Source: CAD feature listing. Evaluate the final solid. Frame: model axes, mm. Face numbers are marked on the shaded views. A direction names the side the tool comes from. Round coordinates to 2 decimals unless told otherwise and drop trailing zeros. Order: outer loops, then holes, each group sorted by start corner. A loop starts at its lowest first (then second) coordinate and runs counter-clockwise, first axis right, second up. Notation, with made-up numbers: (29, -19.75) -> (78, -19.75) arc R11 cw to (78, -4.75) -> close; hole circle Ø7 at (-5.5, -16). An arc over 180 degrees is marked (long way). Answer as CSV lines item,"result".
from build123d import *

# Parameters (mm, degrees)
F1_DEPTH = 1.5
F3_DEPTH = 1.5


with BuildPart() as f1:
    # F0 (on Front) → F1 (new body)
    with BuildSketch(Plane.XZ):
        with BuildLine():
            Line((0, 5), (0, 10))
            Line((0, 10), (-115, 10))
            Line((-115, 10), (-115, -10))
            Line((-115, -10), (0, -10))
            Line((0, -10), (0, -5))
            Line((0, -5), (-50, -5))
            ThreePointArc((-50, -5), (-53.535534, -3.535534), (-55, 0))
            ThreePointArc((-55, 0), (-53.535534, 3.535534), (-50, 5))
            Line((-50, 5), (0, 5))
        make_face()
        with BuildLine():
            ThreePointArc((-65, 0), (-66.464466, -3.535534), (-70, -5))
            Line((-70, -5), (-100, -5))
            ThreePointArc((-100, -5), (-103.535534, -3.535534), (-105, 0))
            ThreePointArc((-105, 0), (-103.535534, 3.535534), (-100, 5))
            Line((-100, 5), (-70, 5))
            ThreePointArc((-70, 5), (-66.464466, 3.535534), (-65, 0))
        make_face(mode=Mode.SUBTRACT)
        with BuildLine():
            Line((0, 0), (0, 5))
            Line((0, 5), (-50, 5))
            ThreePointArc((-50, 5), (-53.535534, 3.535534), (-55, 0))
            ThreePointArc((-55, 0), (-53.535534, -3.535534), (-50, -5))
            Line((-50, -5), (0, -5))
            Line((0, -5), (0, 0))
        make_face()
    extrude(amount=F1_DEPTH)

    # F2 (on face) → F3 (join)
    with BuildSketch(Plane(origin=(-115, 0, 0), x_dir=(0, -1, 0), z_dir=(-1, 0, 0))):
        with BuildLine():
            Line((1.5, -10), (1.5, 10))
            Line((1.5, 10), (-73.5, 10))
            ThreePointArc((-73.5, 10), (-77.035534, 8.535534), (-78.5, 5))
            Line((-78.5, 5), (-78.5, -5))
            ThreePointArc((-78.5, -5), (-77.035534, -8.535534), (-73.5, -10))
            Line((-73.5, -10), (1.5, -10))
        make_face()
        with BuildLine():
            Line((-48.5, -5), (-63.5, -5))
            ThreePointArc((-63.5, -5), (-67.035534, -3.535534), (-68.5, 0))
            ThreePointArc((-68.5, 0), (-67.035534, 3.535534), (-63.5, 5))
            Line((-63.5, 5), (-48.5, 5))
            ThreePointArc((-48.5, 5), (-44.964466, 3.535534), (-43.5, 0))
            ThreePointArc((-43.5, 0), (-44.964466, -3.535534), (-48.5, -5))
        make_face(mode=Mode.SUBTRACT)
    extrude(amount=F3_DEPTH)


solid = f1.part
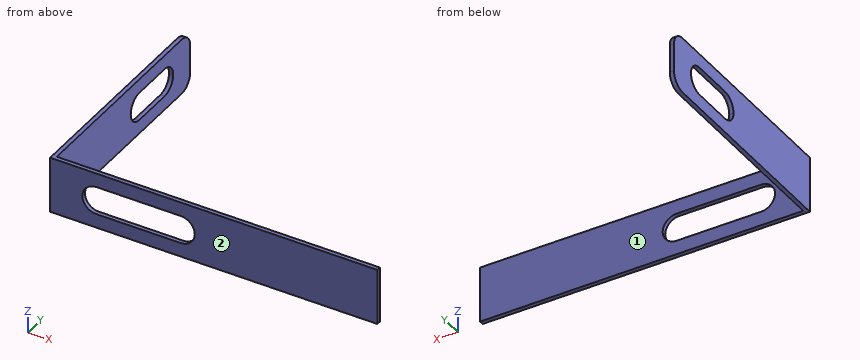
1. Section query A-A on x = -88. Return loops of the section in (y, z).
Results below:
outline,"(-1.5, -10) -> (0, -10) -> (0, -5) -> (-1.5, -5) -> close; (-1.5, 5) -> (0, 5) -> (0, 10) -> (-1.5, 10) -> close"
2. Section query C-C on y = 62. Return loops of the section in (x, z), and give its area (3 significant figures).
Results below:
outline,"(-116.5, -10) -> (-115, -10) -> (-115, -5) -> (-116.5, -5) -> close; (-116.5, 5) -> (-115, 5) -> (-115, 10) -> (-116.5, 10) -> close"
area,"15.0 mm2"
3. Section query D-D on z = 8. Return loops of the section in (x, y).
Results below:
outline,"(-116.5, -1.5) -> (0, -1.5) -> (0, 0) -> (-115, 0) -> (-115, 77.5) -> (-116.5, 77.5) -> close"
4. Line query: L1, parallel to Y at x = -9.5, z = 0.5; L2, parallel to X at y = 23, z = -2. Output: solid intervals per line, ascending. Write a range as [from, to].
Results below:
L1,"[-1.5, 0]"
L2,"[-116.5, -115]"
5. Pin query (flat end, axial travel): pin 1 (6 mm diameter, centred on y = 21, z = 4.5, fed in from +X); pin 2 (1.5 mm diameter, centred on x = -50, z = 2, fed in from +Y). Return the tip coordinate at first contact, or that it passes through.
Results below:
pin 1,"x = -115"
pin 2,"y = 0"
6. Section query B-B on z = 3. Return loops of the section in (x, y).
Results below:
outline,"(-116.5, -1.5) -> (-104, -1.5) -> (-104, 0) -> (-115, 0) -> (-115, 44.5) -> (-116.5, 44.5) -> close; (-116.5, 67.5) -> (-115, 67.5) -> (-115, 78.5) -> (-116.5, 78.5) -> close; (-66, -1.5) -> (0, -1.5) -> (0, 0) -> (-66, 0) -> close"
7. Reachability of the marked faces 1 and 2 from +Z, -Z, +X, -X, +Y, -Y: full face, straight path, thin tool, end or side. Return the list, or none.
Results below:
face 1,"+Z, -Z, +X, +Y"
face 2,"+Z, -Z, +X, -X, -Y"
